The model under review builds one solid part; all positions refer to its coordinate system, in mm. Face numbers are marked on the shaded views. A direction names the side the tool comes from. Give positions to 0.01 mm unless a question says otherwise; leave off trailing zeros. Loops run counter-clockwise (first coordinate to the right, second up) from the corner with the lowest first, then second, coordinate; pieces in that order, holes last. Notation, with made-up numbers: M 43,21 L 99,21 A12 cw 99,32 Z; hole C -3,-21.75 d3. An arc over 180 degrees is marked long. Return JSON: item names as keys, results as strings.
```python
from build123d import *

# Parameters (mm, degrees)
F1_DEPTH = 7
F2_DEPTH = 6
F3_DEPTH = 15


# Not quite as in the source:
# - a feature names something its author has since deleted; it is built from what else it names


with BuildPart() as f1:
    # F0 (on Front) → F1 (new body)
    with BuildSketch(Plane.XZ):
        with BuildLine():
            Line((-3.9138396984, -1.8700768013), (-3.3236176952, -1.6008211246))
            Line((-3.3236176952, -1.6008211246), (-3.3236176952, -2.2903047641))
            Line((-3.3236176952, -2.2903047641), (-2.590710345, -2.2903047641))
            Line((-2.590710345, -2.2903047641), (-2.590710345, -3.7436034497))
            Line((-2.590710345, -3.7436034497), (-2.1779115118, -2.7734910012))
            ThreePointArc((-2.1779115118, -2.7734910012), (-0.2255882059, 2.7885019734), (2.7665772748, -2.2903047641))
            Line((2.7665772748, -2.2903047641), (3.4491920394, -2.2903047641))
            Line((3.4491920394, -2.2903047641), (3.4491920394, -1.6408955531))
            Line((3.4491920394, -1.6408955531), (4.0849162776, -1.8976975874))
            ThreePointArc((4.0849162776, -1.8976975874), (4.3385221106, -0.3163391945), (3.988877441, 1.2465935905))
            Line((3.988877441, 1.2465935905), (5.5865912817, 3.465253188))
            Line((5.5865912817, 3.465253188), (5.5865912817, 5.931237081))
            Line((5.5865912817, 5.931237081), (1.5955031972, 5.931237081))
            Line((1.5955031972, 5.931237081), (4.5903746292, 3.397220974))
            Line((4.5903746292, 3.397220974), (0.0905031972, 3.431237081))
            Line((0.0905031972, 3.431237081), (-4.4093682348, 3.465253188))
            Line((-4.4093682348, 3.465253188), (-1.4144968028, 5.931237081))
            Line((-1.4144968028, 5.931237081), (-5.4144968028, 5.931237081))
            Line((-5.4144968028, 5.931237081), (-5.4144968028, 3.465253188))
            Line((-5.4144968028, 3.465253188), (-3.8254308087, 1.2055638243))
            ThreePointArc((-3.8254308087, 1.2055638243), (-4.1577420716, -0.3239748955), (-3.9138396984, -1.8700768013))
        make_face()
        Polygon((-3.3236176952, -2.2903047641), (-3.3236176952, -1.6008211246), (-3.9138396984, -1.8700768013), (-4.090710345, -1.9507641112), (-4.090710345, -2.2903047641), align=None)
        Polygon((-2.590710345, -2.2903047641), (-3.3236176952, -2.2903047641), (-4.090710345, -2.2903047641), (-4.090710345, -4.9565606735), (-3.3236176952, -4.9565606735), (-2.590710345, -4.9565606735), (-2.590710345, -3.7436034497), align=None)
        with BuildLine():
            Line((3.4491920394, -2.2903047641), (2.7665772748, -2.2903047641))
            ThreePointArc((2.7665772748, -2.2903047641), (2.7416681899, -2.3259370036), (2.7162846892, -2.3612328517))
            Line((2.7162846892, -2.3612328517), (2.7162846892, -3.7879117456))
            Line((2.7162846892, -3.7879117456), (2.7162846892, -4.9565606735))
            Line((2.7162846892, -4.9565606735), (4.2162846892, -4.9497258588))
            Line((4.2162846892, -4.9497258588), (4.2162846892, -2.2903047641))
            Line((4.2162846892, -2.2903047641), (3.4491920394, -2.2903047641))
        make_face()
        with BuildLine():
            ThreePointArc((2.7162846892, -2.3612328517), (2.7416681899, -2.3259370036), (2.7665772748, -2.2903047641))
            Line((2.7665772748, -2.2903047641), (2.7162846892, -2.3612328517))
        make_face()
        Polygon((1.5955031972, 5.931237081), (-1.4144968028, 5.931237081), (-4.4093682348, 3.465253188), (0.0905031972, 3.431237081), (4.5903746292, 3.397220974), align=None)
        with BuildLine():
            Line((2.7162846892, -3.7879117456), (2.7162846892, -2.3612328517))
            ThreePointArc((2.7162846892, -2.3612328517), (2.5117247114, -2.6140814767), (2.2829176272, -2.8452189465))
            Line((2.2829176272, -2.8452189465), (2.7162846892, -3.7879117456))
        make_face()
        Polygon((3.4491920394, -1.6408955531), (3.4491920394, -2.2903047641), (4.2162846892, -2.2903047641), (4.2162846892, -1.9507641112), (4.0849162776, -1.8976975874), align=None)
    extrude(amount=F1_DEPTH)

    # F0 (on Front) → F2 (cut)
    with BuildSketch(Plane.XZ):
        Polygon((1.5955031972, 5.931237081), (-1.4144968028, 5.931237081), (-4.4093682348, 3.465253188), (0.0905031972, 3.431237081), (4.5903746292, 3.397220974), align=None)
    extrude(amount=F2_DEPTH, mode=Mode.SUBTRACT)

    # F0 (on Front) → F3 (join)
    with BuildSketch(Plane.XZ):
        Polygon((-2.590710345, -2.2903047641), (-3.3236176952, -2.2903047641), (-4.090710345, -2.2903047641), (-4.090710345, -4.9565606735), (-3.3236176952, -4.9565606735), (-2.590710345, -4.9565606735), (-2.590710345, -3.7436034497), align=None)
        with BuildLine():
            Line((3.4491920394, -2.2903047641), (2.7665772748, -2.2903047641))
            ThreePointArc((2.7665772748, -2.2903047641), (2.7416681899, -2.3259370036), (2.7162846892, -2.3612328517))
            Line((2.7162846892, -2.3612328517), (2.7162846892, -3.7879117456))
            Line((2.7162846892, -3.7879117456), (2.7162846892, -4.9565606735))
            Line((2.7162846892, -4.9565606735), (4.2162846892, -4.9497258588))
            Line((4.2162846892, -4.9497258588), (4.2162846892, -2.2903047641))
            Line((4.2162846892, -2.2903047641), (3.4491920394, -2.2903047641))
        make_face()
    extrude(amount=-F3_DEPTH)


solid = f1.part
```
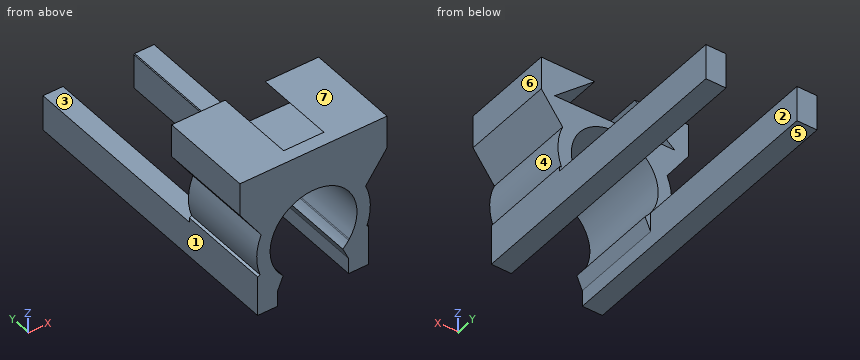
1) Consider section D-D on z = 5.25. Write out the cut boundary in (x, y).
From the geometry:
{"outline": "M -5.41,-7 L 5.59,-7 L 5.59,0 L 2.4,0 L 2.4,-6 L -2.24,-6 L -2.24,0 L -5.41,0 Z"}
2) Insertion check: pin 1 (4 mm diameter, centred on x = 1.5, y = -4, fed in from +Z); pin 2 (0.8 mm diameter, centred on y = 7.5, z = -3.5, fed in from -X); pin 3 (0.7 mm diameter, centred on x = 3, y = 9.5, fed in from +Z); pin 4 (2 mm diameter, centred on y = 9.5, z = -3.5, fed in from +X). Each pin has a flat end and moves straight along its axis. Give the tip position at first contact, or say it passes through.
From the geometry:
{"pin 1": "z = 5.93", "pin 2": "x = -4.09", "pin 3": "z = -2.29", "pin 4": "x = 4.22"}
3) Consider section A-A on y = 9.25. Write out the cut boundary in (x, z), then the cut area to 3 significant figures.
From the geometry:
{"outline": "M -4.09,-4.96 L -2.59,-4.96 L -2.59,-2.29 L -4.09,-2.29 Z; M 2.72,-4.96 L 4.22,-4.95 L 4.22,-2.29 L 2.77,-2.29 A3.25 cw 2.72,-2.36 Z", "area": "7.99 mm²"}
4) Consider section B-B on z = -1.5. Write out the cut boundary in (x, y), then the cut area to 3 significant figures.
From the geometry:
{"outline": "M -4.03,-7 L -2.98,-7 L -2.98,0 L -4.03,0 Z; M 3.16,-7 L 4.21,-7 L 4.21,0 L 3.16,0 Z", "area": "14.6 mm²"}
5) The part is to be moulded in two halves that separate along Z. For the marked faces 4, 5, 6 and 7, say which applies: released by +Z, released by -Z, zero draft, split by the parting line, or undercut.
From the geometry:
{"face 4": "undercut", "face 5": "released by -Z", "face 6": "zero draft", "face 7": "released by +Z"}
6) Wall thickness on L1, parallel to X at y = -4.25, z = -0.5; L2, parallel to X at y = 10.25, z = -4.5; L3, parallel to Y at x = -1.25, z = 3.25: over which ranges is each line inside the solid? List them lowest first. Write a range as from..to.
From the geometry:
{"L1": "-4.16..-3.16, 3.34..4.34", "L2": "-4.09..-2.59, 2.72..4.22", "L3": "-7..0"}
7) Consider section C-C on y = -1.75. Write out the cut boundary in (x, z).
From the geometry:
{"outline": "M -5.41,3.47 L -3.83,1.21 A4.25 ccw -3.91,-1.87 L -4.09,-1.95 L -4.09,-4.96 L -2.59,-4.96 L -2.59,-3.74 L -2.18,-2.77 A3.25 cw long 2.77,-2.29 L 2.72,-2.36 A3.25 cw 2.28,-2.85 L 2.72,-3.79 L 2.72,-4.96 L 4.22,-4.95 L 4.22,-1.95 L 4.08,-1.9 A4.25 ccw 3.99,1.25 L 5.59,3.47 L 5.59,5.93 L 1.6,5.93 L 4.59,3.4 L -4.41,3.47 L -1.41,5.93 L -5.41,5.93 Z"}
8) Tool access review of the marked faces 1, 2 and 3: name each direction out of +Z, -Z, +X, -X, +Y, -Y from which nothing blocks a thin tool from reaching the whole face with its end or side.
From the geometry:
{"face 1": "-Z, -X, +Y, -Y", "face 2": "-Z, +Y", "face 3": "+Z, +X, -X, +Y"}
